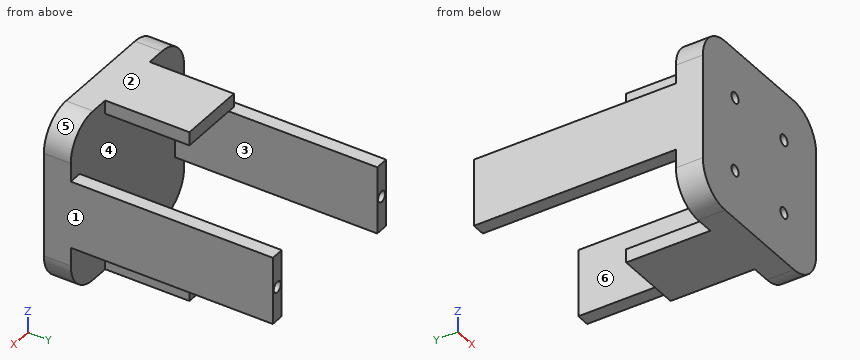
```python
from build123d import *

# Parameters (mm, degrees)
ESBO_O1_W                = 51
ESBO_O1_H                = 51
RESSALTO_EXTRUS_O1_DEPTH = 8
ESBO_O2_W                = 4
ESBO_O2_H                = 20
RESSALTO_EXTRUS_O2_DEPTH = 60
ESBO_O3_R                = 1.6
CORTE_EXTRUS_O1_DEPTH    = 7
ESBO_O4_W                = 20
ESBO_O4_H                = 4
RESSALTO_EXTRUS_O3_DEPTH = 25
ESBO_O5_R                = 1.6
CORTE_EXTRUS_O2_DEPTH    = 7
FILETE2_R                = 10


with BuildPart() as part:
    # Esboço1 → Ressalto-extrusão1 (new body)
    with BuildSketch(Plane(origin=(0, 0, 0), x_dir=(1, 0, 0), z_dir=(0, 1, 0))):
        Rectangle(ESBO_O1_W, ESBO_O1_H)
    extrude(amount=RESSALTO_EXTRUS_O1_DEPTH)

    # Esboço2 → Ressalto-extrusão2 (add)
    with BuildSketch(Plane(origin=(0, 8, 0), x_dir=(1, 0, 0), z_dir=(0, 1, 0))):
        with Locations((-23.5, 0)):
            Rectangle(ESBO_O2_W, ESBO_O2_H)
        with Locations((23.5, 0)):
            Rectangle(ESBO_O2_W, ESBO_O2_H)
    extrude(amount=RESSALTO_EXTRUS_O2_DEPTH)

    # Esboço3 → Corte-extrusão1 (cut)
    with BuildSketch(Plane(origin=(0, 68, 0), x_dir=(1, 0, 0), z_dir=(0, 1, 0))):
        with Locations(Location((-23.5, 0, 0), (0, 0, 270))):
            Circle(ESBO_O3_R)
        with Locations(Location((23.5, 0, 0), (0, 0, 90))):
            Circle(ESBO_O3_R)
    extrude(amount=-CORTE_EXTRUS_O1_DEPTH, mode=Mode.SUBTRACT)

    # Esboço4 → Ressalto-extrusão3 (add)
    with BuildSketch(Plane(origin=(0, 8, 0), x_dir=(1, 0, 0), z_dir=(0, 1, 0))):
        with Locations((0, 23.5)):
            Rectangle(ESBO_O4_W, ESBO_O4_H)
        with Locations((0, -23.5)):
            Rectangle(ESBO_O4_W, ESBO_O4_H)
    extrude(amount=RESSALTO_EXTRUS_O3_DEPTH)

    # Esboço5 → Corte-extrusão2 (cut)
    with BuildSketch(Plane.XZ):
        with Locations(Location((-11, 11, 0), (0, 0, 270))):
            Circle(ESBO_O5_R)
        with Locations(Location((11, 11, 0), (0, 0, 90))):
            Circle(ESBO_O5_R)
        with Locations(Location((11, -11, 0), (0, 0, 270))):
            Circle(ESBO_O5_R)
        with Locations(Location((-11, -11, 0), (0, 0, 90))):
            Circle(ESBO_O5_R)
    extrude(amount=-CORTE_EXTRUS_O2_DEPTH, mode=Mode.SUBTRACT)

    # Filete2
    filete2_edges = [part.edges().sort_by_distance(p)[0] for p in [
        (25.5, 4, 25.5),
        (-25.5, 4, 25.5),
        (-25.5, 4, -25.5),
        (25.5, 4, -25.5),
    ]]
    fillet(filete2_edges, radius=FILETE2_R)


solid = part.part
```
CAD build for the part. Positions are in the model's coordinates, mm. Face numbers are marked on the shaded views. A direction names the side the tool comes from. Round coordinates to 2 decimals unless told otherwise and drop trailing zeros. Write each loop counter-clockwise with the first axis right and the second up, starting at its lowest first coordinate (ties: lowest second). Pieces come first, ordered by that corner, then holes.
Item 1: Mould opens along X. For the marked faces 1, 2 and 3 say: released by +X, released by -X, zero draft, split by the parting line, or undercut.
Filled in:
face 1: released by +X
face 2: zero draft
face 3: undercut
Item 2: Band-saw the part on C-C on y = 44. Write the cut outline in (x, z), then the cut area to 3 significant figures.
Filled in:
outline: (-25.5, -10) - (-21.5, -10) - (-21.5, 10) - (-25.5, 10) - close; (21.5, -10) - (25.5, -10) - (25.5, 10) - (21.5, 10) - close
area: 160 mm2
Item 3: Tool access for the marked faces 4, 5 and 6: list every direction of +Z, -Z, +X, -X, +Y, -Y with a clear straight run to the whole face (end or side of a thin tool).
Filled in:
face 4: +Y
face 5: +Z, +X, +Y, -Y
face 6: +Z, -Z, +Y
Item 4: Band-saw the part on A-A on y = 24. Write the cut outline in (x, z).
Filled in:
outline: (-25.5, -10) - (-21.5, -10) - (-21.5, 10) - (-25.5, 10) - close; (-10, -25.5) - (10, -25.5) - (10, -21.5) - (-10, -21.5) - close; (-10, 21.5) - (10, 21.5) - (10, 25.5) - (-10, 25.5) - close; (21.5, -10) - (25.5, -10) - (25.5, 10) - (21.5, 10) - close
Item 5: Band-saw the part on D-D on z = -5. Write the cut outline in (x, y).
Filled in:
outline: (-25.5, 0) - (25.5, 0) - (25.5, 68) - (21.5, 68) - (21.5, 8) - (-21.5, 8) - (-21.5, 68) - (-25.5, 68) - close
Item 6: Band-saw the part on B-B on x = -11. Write the cut outline in (y, z), then the cut area to 3 significant figures.
Filled in:
outline: (0, -25.5) - (8, -25.5) - (8, 25.5) - (0, 25.5) - (0, 12.6) - (7, 12.6) - (7, 9.4) - (0, 9.4) - (0, -9.4) - (7, -9.4) - (7, -12.6) - (0, -12.6) - close
area: 363 mm2
Item 7: Drill centre lines: L1, parallel to X at y = 3, z = 11; L2, parallel to Z at x = 23.5, y = 66.5; L3, parallel to X at y = 57, z = 3. Where is each one in solid material? Low to high.
Filled in:
L1: x = -25.5 to -12.6, -9.4 to 9.4, 12.6 to 25.5
L2: z = -10 to -1.6, 1.6 to 10
L3: x = -25.5 to -21.5, 21.5 to 25.5
Item 8: Drop flat-ended pins along their axis: pin 1 Ø3 at (x, z) = (11, -11) entering from +Y; pin 2 Ø5 at (x, y) = (-13.5, 18.5) entering from +Z; pin 3 Ø2 at (y, z) = (16.5, 23) entering from +X; pin 4 Ø3 at (x, y) = (-23.5, 36.5) entering from -Z. Give the stop position or say it passes through.
Filled in:
pin 1: stops at y = 8
pin 2: passes through
pin 3: stops at x = 10
pin 4: stops at z = -10
